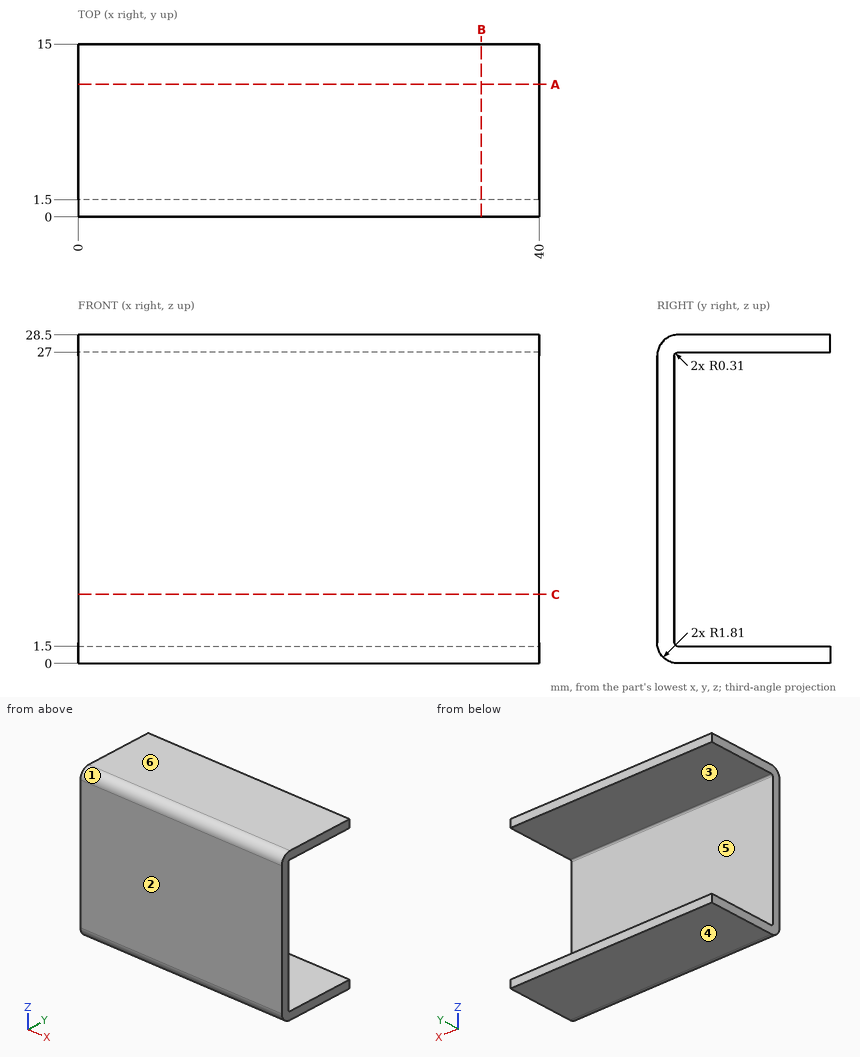
Here's the drawing with two shaded views (mm, measured from the low corner). I have some questions. A direction names the side the tool comes from. Give positions to 0.01 mm unless a question says otherwise; leave off trailing zeros. Loops run counter-clockwise (first coordinate to the right, second up) from the corner with the lowest first, then second, coordinate; pieces in that order, holes last. Notation, with made-up numbers: (-10, -10) - (38, -10) arc R33 cw to (38, 20) - close; hole circle Ø9 at (-6, -36). An arc over 180 degrees is marked (long way). One line per item, written item: value.
(1) On a 3-axis mill with a long thin cutter (end or side, diameter ignored), from which of +Z, -Z, +X, -X, +Y, -Y can I reach the whole of each face in a straight line? I mean the marked faces 5 and 6. Say none if no direction works.
Verdict:
face 5: +X, -X, +Y
face 6: +Z, +X, -X, +Y, -Y
(2) If we mould it in two halves opening along Z, with no side actions, what happens to the marked faces 1, 2, 3 and 4? For each: released by +Z, released by -Z, zero draft, split by the parting line, or undercut.
Verdict:
face 1: released by +Z
face 2: zero draft
face 3: undercut
face 4: released by -Z
(3) If we section it at B-B, the plane x = 35: List the corners of the cut face in (y, z) for me.
Verdict:
outline: (0, 1.81) arc R1.81 ccw to (1.81, 0) - (15, 0) - (15, 1.5) - (1.81, 1.5) arc R0.31 cw to (1.5, 1.81) - (1.5, 26.69) arc R0.31 cw to (1.81, 27) - (15, 27) - (15, 28.5) - (1.81, 28.5) arc R1.81 ccw to (0, 26.69) - close
(4) If we section it at A-A, the plane y = 11.5: List the corners of the cut face in (x, z) for me.
Verdict:
outline: (0, 0) - (40, 0) - (40, 1.5) - (0, 1.5) - close; (0, 27) - (40, 27) - (40, 28.5) - (0, 28.5) - close
(5) I need wall thicknesses on line 1 along Z through (x, y) = (4, 7.5); line 2 along Y through (x, z) = (25, 19.5); line 3 along Z through (x, y) = (30.5, 1). Which ranges of each line are inside material? Lowest first, please.
Verdict:
line 1: 0 to 1.5, 27 to 28.5
line 2: 0 to 1.5
line 3: 0.19 to 28.31
(6) If we section it at C-C, the plane z = 6: List the corners of the cut face in (x, y) for me, plus the area to 3 significant figures.
Verdict:
outline: (0, 0) - (40, 0) - (40, 1.5) - (0, 1.5) - close
area: 60.0 mm^2
(7) I'm going to push flat-ended pins straight in: pin 1 (6 mm diameter, centred on x = 6, y = 6.5, fed in from -Z); pin 2 (7.5 mm diameter, centred on x = 17, z = 16, fed in from +Y). Where does each tip first touch, or does it pass through?
Verdict:
pin 1: z = 0
pin 2: y = 1.5
